Design review of the part built by this model. Coordinates are the model's own, in mm. Give positions to 0.01 mm unless a question says otherwise; leave off trailing zeros. Loops run counter-clockwise (first coordinate to the right, second up) from the corner with the lowest first, then second, coordinate; pieces in that order, holes last. Notation, with made-up numbers: (69, 34.25) - (78, 34.25) arc R23 ccw to (78, 48.25) - close; hole circle Ø3 at (-29.5, 40.25). An arc over 180 degrees is marked (long way). Write each question's results on one line, items separated by ' | '.
Solid Edge part; units mm, degrees
sketch "Sketch1" plane through (0, 0, 0) normal (1, 0, 0) x (0, 1, 0)
  line L0 (59.8954, 25.3571) -> (0, 25.3571)
  line L1 (0, 25.3571) -> (0, 17.5785)
  line L2 (0, 17.5785) -> (3, 17.5785)
  line L3 (3, 17.5785) -> (3, 7.7785)
  line L4 (3, 7.7785) -> (0, 7.7785)
  line L5 (0, 7.7785) -> (0, 0)
  line L6 (0, 0) -> (5.0714, -10.8757)
  line L7 (5.0714, -10.8757) -> (63.9814, 16.5945)
  line L8 (62.1005, 20.6281) -> (63.9814, 16.5945)
  line L9 (59.3816, 19.3602) -> (62.1005, 20.6281)
  line L10 (57.3953, 23.6198) -> (59.3816, 19.3602)
  line L11 (60.1142, 24.8877) -> (57.3953, 23.6198)
  line L12 (59.8954, 25.3571) -> (60.1142, 24.8877)
  dimension "D1" = 3
  dimension "D2" = 5.0714
  dimension "D3" = 57.3953
  dimension "D4" = 62.1005
extrude "Protrusion1" add sketch "Sketch1" against normal blind 3
sketch "Sketch2" plane through (0, 0, 0) normal (0, -1, 0) x (1, 0, 0)
  line L0 (-8.2565, 24.3571) -> (6.8913, 24.3571)
extrude "Cutout1" cut sketch "Sketch2" against normal through all material side at (-0.6826, 0, 24.4071)
properties material "Acier"
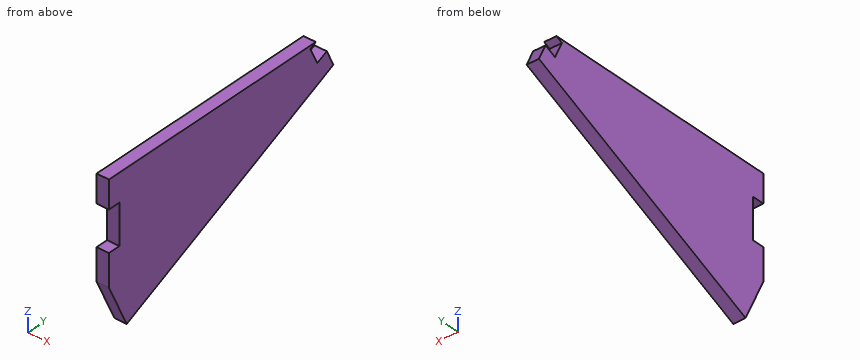
(1) Take a section at B-B on y = 25.5. Give the boundary of the cut face in (x, z), plus the area to 3 significant figures.
Answers below:
outline: (-3, -1.35) - (0, -1.35) - (0, 24.36) - (-3, 24.36) - close | area: 77.1 mm2
(2) Insertion check: P1, Ø1, axis at y = 9.5, z = 4, coming from the +X side. The pin has a flat end and moves straight along its axis. Give the tip position at first contact, or say it passes through.
Answers below:
P1: x = 0
(3) Take a section at C-C on z = 14.5. Give the boundary of the cut face in (x, y).
Answers below:
outline: (-3, 3) - (0, 3) - (0, 59.49) - (-3, 59.49) - close
(4) Take a section at A-A on x = -1.1. Give the boundary of the cut face in (y, z).
Answers below:
outline: (0, 0) - (5.07, -10.88) - (63.98, 16.59) - (62.1, 20.63) - (59.38, 19.36) - (57.4, 23.62) - (58.98, 24.36) - (0, 24.36) - (0, 17.58) - (3, 17.58) - (3, 7.78) - (0, 7.78) - close
(5) Wall thickness on line 1 along Y through (x, z) = (-0.9, 0.5); line 2 along Y through (x, z) = (-2.15, -7.5); line 3 along Z through (x, y) = (-1.35, 44.5): over which ranges is each line inside the solid? List them lowest first. Write a range as from..to.
Answers below:
line 1: 0..29.47 | line 2: 3.5..12.31 | line 3: 7.51..24.36
